```python
from build123d import *

# Parameters (mm, degrees)
SKETCH1_R           = 50.8
SKETCH1_R_2         = 2.9
BOSS_EXTRUDE1_DEPTH = 6.35
SKETCH2_R           = 25.4
BOSS_EXTRUDE2_DEPTH = 12.7
SKETCH3_R           = 12.7
CUT_EXTRUDE1_DEPTH  = 12.7


with BuildPart() as part:
    # Sketch1 → Boss-Extrude1 (new body)
    with BuildSketch(Plane(origin=(0, 0, 0), x_dir=(0, 0, -1), z_dir=(1, 0, 0))):
        with Locations((0, 0.711302035)):
            Circle(SKETCH1_R)
        with Locations((-36.235253271, 12.484849521)):
            Circle(SKETCH1_R_2, mode=Mode.SUBTRACT)
        with Locations((-22.394618112, -30.112245451)):
            Circle(SKETCH1_R_2, mode=Mode.SUBTRACT)
        with Locations((22.394618112, -30.112245451)):
            Circle(SKETCH1_R_2, mode=Mode.SUBTRACT)
        with Locations((36.235253271, 12.484849521)):
            Circle(SKETCH1_R_2, mode=Mode.SUBTRACT)
        with Locations((0, 38.811302035)):
            Circle(SKETCH1_R_2, mode=Mode.SUBTRACT)
    extrude(amount=BOSS_EXTRUDE1_DEPTH)

    # Sketch2 → Boss-Extrude2 (add)
    with BuildSketch(Plane(origin=(6.35, 0, 0), x_dir=(0, 0, -1), z_dir=(1, 0, 0))):
        Circle(SKETCH2_R)
    extrude(amount=BOSS_EXTRUDE2_DEPTH)

    # Sketch3 → Cut-Extrude1 (cut)
    with BuildSketch(Plane(origin=(19.05, 0, 0), x_dir=(0, 0, -1), z_dir=(1, 0, 0))):
        Circle(SKETCH3_R)
    extrude(amount=-CUT_EXTRUDE1_DEPTH, mode=Mode.SUBTRACT)


solid = part.part
```
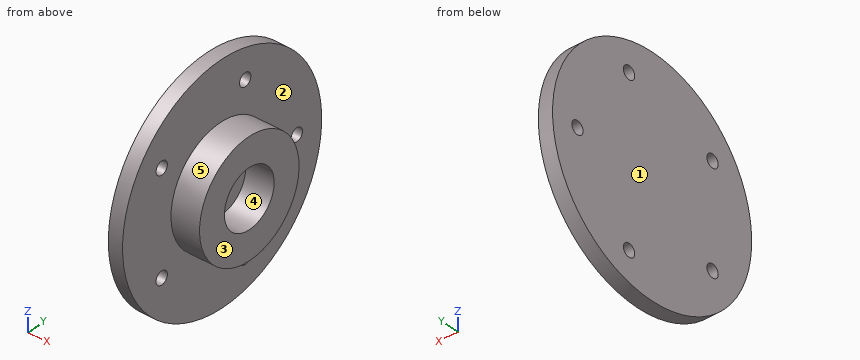
Input: part model. Units: mm. Frame: model coordinates. Face numbers are marked on the shaded views. A direction names the side the tool comes from. Round coordinates to 2 decimals unless told otherwise and drop trailing zeros. Loops run counter-clockwise (first coordinate to the right, second up) from the corner with the lowest first, then second, coordinate; pieces in that order, holes last. Notation, with made-up numbers: M 31.25,75.25 L 59.25,75.25 A13 ccw 59.25,85.25 Z; hole C -19.75,47 d1. An arc over 180 degrees is marked long. Answer in a Markdown table with one row per item. Add a question column.
1. Ray query, probe 1 along X at (y, z) = (-38, 19); probe 2 along Z at (x, y) = (7.75, -10.5); probe 3 along Y at (x, z) = (4, 35.5). Return the intervals inside material, ascending.
2. Contact query for flat-ended pins moving along their axis: pin 1 (8 mm diameter, centred on x = 9, y = -23, fed in from -Z); pin 2 (4 mm diameter, centred on x = 6, y = -26, fed in from -Z); pin 3 (6.5 mm diameter, centred on y = 12.48, z = -36.24, fed in from +X). Output: stop coordinate, or through.
3. Mould query, pull axis Z, two halves, no side actions, for the marked faces 3, 4 and 5. Classes: released by +Z, released by -Z, zero draft, split by the parting line, or undercut.
4. Section A-A (z = 0). Output: boundary loops of the cut face in (x, y).
5. Section C-C (x = 15.5). Output: boundary loops of the cut face in (y, z).
6. Section B-B (y = 40.5). Output: boundary loops of the cut face in (x, z), and give its area (3 significant figures).
7. Section D-D (x = 4.75). Output: boundary loops of the cut face in (y, z).
8. Set-up query: the marked faces 1 and 2. Return all of +Z, -Z, +X, -X, +Y, -Y with unobstructed straight access to the full face (end or side cutting, diameter ignored); none if empty.
Values follow:
| question | item | result |
|---|---|---|
| 1 | probe 1 | 0 to 6.35 |
| 1 | probe 2 | -23.13 to -7.14, 7.14 to 23.13 |
| 1 | probe 3 | -35.63 to 9.68, 15.29 to 37.05 |
| 2 | pin 1 | z = -46.38 |
| 2 | pin 2 | z = -44.38 |
| 2 | pin 3 | x = 6.35 |
| 3 | face 3 | zero draft |
| 3 | face 4 | undercut |
| 3 | face 5 | split by the parting line |
| 4 | outline | M 0,-50.09 L 6.35,-50.09 L 6.35,-25.4 L 19.05,-25.4 L 19.05,-12.7 L 6.35,-12.7 L 6.35,12.7 L 19.05,12.7 L 19.05,25.4 L 6.35,25.4 L 6.35,35.91 L 0,35.91 Z; M 0,41.71 L 6.35,41.71 L 6.35,51.51 L 0,51.51 Z |
| 5 | outline | C 0,0 d50.8; hole C 0,0 d25.4 |
| 6 | outline | M 0,-31.58 L 6.35,-31.58 L 6.35,-2.36 L 0,-2.36 Z; M 0,2.36 L 6.35,2.36 L 6.35,31.58 L 0,31.58 Z |
| 6 | area | 371 mm^2 |
| 7 | outline | C 0.71,0 d101.6; hole C -30.11,-22.39 d5.8; hole C -30.11,22.39 d5.8; hole C 12.48,-36.24 d5.8; hole C 12.48,36.24 d5.8; hole C 38.81,0 d5.8 |
| 8 | face 1 | +Z, -Z, -X, +Y, -Y |
| 8 | face 2 | +X |
